CAD build for the part. Positions are in the model's coordinates, mm. A direction names the side the tool comes from. Round coordinates to 2 decimals unless told otherwise and drop trailing zeros. Loops run counter-clockwise (first coordinate to the right, second up) from the corner with the lowest first, then second, coordinate; pieces in that order, holes last. Notation, with made-up numbers: (86.25, 27) - (106.25, 27) arc R21 cw to (106.25, 53) - close; hole circle Ø2 at (-31, 31). An arc over 180 degrees is marked (long way). Use one line per item in the form item = value.
from build123d import *

# Parameters (mm, degrees)
BOSS_EXTRUDE1_DEPTH = 20
FILLET1_R           = 2
CUT_EXTRUDE1_DEPTH  = 76.381086892
CHAMFER1_SIZE       = 0.5
CHAMFER2_SIZE       = 10
CHAMFER3_SIZE       = 1


with BuildPart() as part:
    # Sketch1 → Boss-Extrude1 (new body)
    with BuildSketch(Plane.XY):
        with BuildLine():
            Line((12.7, 20.547), (-12.7, 20.547))
            ThreePointArc((-12.7, 20.547), (-27.228923033, 14.528923033), (-33.247, 0))
            Line((-33.247, 0), (-33.247, -20.447))
            Line((-33.247, -20.447), (-60.015, -20.447))
            Line((-60.015, -20.447), (-60.015, -16.447))
            Line((-60.015, -16.447), (-37.247, -16.447))
            Line((-37.247, -16.447), (-37.247, 0))
            ThreePointArc((-37.247, 0), (-30.057350158, 17.357350158), (-12.7, 24.547))
            Line((-12.7, 24.547), (12.7, 24.547))
            ThreePointArc((12.7, 24.547), (30.057350158, 17.357350158), (37.247, 0))
            Line((37.247, 0), (37.247, -16.447))
            Line((37.247, -16.447), (60.015, -16.447))
            Line((60.015, -16.447), (60.015, -20.447))
            Line((60.015, -20.447), (33.247, -20.447))
            Line((33.247, -20.447), (33.247, 0))
            ThreePointArc((33.247, 0), (27.228923033, 14.528923033), (12.7, 20.547))
        make_face()
    extrude(amount=BOSS_EXTRUDE1_DEPTH)

    # Fillet1
    fillet1_edges = [part.edges().sort_by_distance(p)[0] for p in [
        (60.015, -18.447, 20),
        (-60.015, -18.447, 0),
        (60.015, -18.447, 0),
        (-60.015, -18.447, 20),
    ]]
    fillet(fillet1_edges, radius=FILLET1_R)

    # Sketch3 → Cut-Extrude1 (cut, through all)
    with BuildSketch(Plane(origin=(0, -16.447, 0), x_dir=(1, 0, 0), z_dir=(0, 1, 0))):
        with BuildLine():
            Line((52.015, -2.4), (56.015, -2.4))
            ThreePointArc((56.015, -2.4), (57.615, -4), (56.015, -5.6))
            Line((56.015, -5.6), (52.015, -5.6))
            ThreePointArc((52.015, -5.6), (50.415, -4), (52.015, -2.4))
        make_face()
        with BuildLine():
            Line((56.015, -17.6), (52.015, -17.6))
            ThreePointArc((52.015, -17.6), (50.415, -16), (52.015, -14.4))
            Line((52.015, -14.4), (56.015, -14.4))
            ThreePointArc((56.015, -14.4), (57.615, -16), (56.015, -17.6))
        make_face()
        with BuildLine():
            Line((-52.015, -5.6), (-56.015, -5.6))
            ThreePointArc((-56.015, -5.6), (-57.615, -4), (-56.015, -2.4))
            Line((-56.015, -2.4), (-52.015, -2.4))
            ThreePointArc((-52.015, -2.4), (-50.415, -4), (-52.015, -5.6))
        make_face()
        with BuildLine():
            Line((-56.015, -14.4), (-52.015, -14.4))
            ThreePointArc((-52.015, -14.4), (-50.415, -16), (-52.015, -17.6))
            Line((-52.015, -17.6), (-56.015, -17.6))
            ThreePointArc((-56.015, -17.6), (-57.615, -16), (-56.015, -14.4))
        make_face()
    extrude(amount=-CUT_EXTRUDE1_DEPTH, mode=Mode.SUBTRACT)

    # Chamfer1
    chamfer1_edges = [part.edges().sort_by_distance(p)[0] for p in [
        (-50.415, -20.447, 16),
        (-54.015, -20.447, 17.6),
        (-57.615, -20.447, 16),
        (-54.015, -20.447, 14.4),
        (-50.415, -16.447, 16),
        (-54.015, -16.447, 14.4),
        (-57.615, -16.447, 16),
        (-54.015, -16.447, 17.6),
        (50.415, -20.447, 4),
        (54.015, -20.447, 2.4),
        (57.615, -20.447, 4),
        (54.015, -20.447, 5.6),
        (50.415, -16.447, 4),
        (54.015, -16.447, 5.6),
        (57.615, -16.447, 4),
        (54.015, -16.447, 2.4),
        (57.615, -20.447, 16),
        (54.015, -20.447, 17.6),
        (50.415, -20.447, 16),
        (54.015, -20.447, 14.4),
        (57.615, -16.447, 16),
        (54.015, -16.447, 14.4),
        (50.415, -16.447, 16),
        (54.015, -16.447, 17.6),
        (-50.415, -20.447, 4),
        (-54.015, -20.447, 5.6),
        (-57.615, -20.447, 4),
        (-54.015, -20.447, 2.4),
        (-50.415, -16.447, 4),
        (-54.015, -16.447, 2.4),
        (-57.615, -16.447, 4),
        (-54.015, -16.447, 5.6),
    ]]
    chamfer(chamfer1_edges, length=CHAMFER1_SIZE)

    # Chamfer2
    chamfer2_edges = [part.edges().sort_by_distance(p)[0] for p in [
        (-37.247, -16.447, 10),
        (37.247, -16.447, 10),
    ]]
    chamfer(chamfer2_edges, length=CHAMFER2_SIZE)

    # Chamfer3
    chamfer3_edges = [part.edges().sort_by_distance(p)[0] for p in [
        (0, 20.547, 0),
        (-27.228923033, 14.528923033, 0),
        (-33.247, -10.2235, 0),
        (33.247, -10.2235, 0),
        (27.228923033, 14.528923033, 0),
        (27.228923033, 14.528923033, 20),
        (-33.247, -10.2235, 20),
        (-27.228923033, 14.528923033, 20),
        (0, 20.547, 20),
        (33.247, -10.2235, 20),
    ]]
    chamfer(chamfer3_edges, length=CHAMFER3_SIZE)


solid = part.part
1) Slice it at D-D (x = 44). Write the cut outline in (y, z), plus the area to 3 significant figures.
Report:
outline = (-20.45, 0) - (-13.2, 0) - (-13.2, 20) - (-20.45, 20) - close
area = 145 mm^2
2) Slice it at B-B (y = -14.5). Write the cut outline in (x, z), plus the area to 3 significant figures.
Report:
outline = (-45.3, 0) - (-34.25, 0) - (-33.25, 1) - (-33.25, 19) - (-34.25, 20) - (-45.3, 20) - close; (33.25, 1) - (34.25, 0) - (45.3, 0) - (45.3, 20) - (34.25, 20) - (33.25, 19) - close
area = 480 mm^2
3) Slice it at C-C (y = -9). Write the cut outline in (x, z).
Report:
outline = (-39.8, 0) - (-34.25, 0) - (-33.25, 1) - (-33.25, 19) - (-34.25, 20) - (-39.8, 20) - close; (33.25, 1) - (34.25, 0) - (39.8, 0) - (39.8, 20) - (34.25, 20) - (33.25, 19) - close
4) Two-plate mould, pull along X, no slides. Class faces 1 (the cylindrical face through (-59.445, -18.419, 0.601)), 2 (the flat face through (-54, -16.447, 10)), 3 (the cylindrical face through (59.445, -18.475, 19.399)), 4 (the conical face through (50.28, -16.81, 16.04)): +X half, -X half, draft (parallel to the pull), parting line (faces both ways), or undercut.
Report:
face_1 = -X half
face_2 = draft
face_3 = +X half
face_4 = undercut
5) Tool access for faces 5 (the conical face through (-27.19, 14.81, 19.17)), 6 (the flat face through (54, -18, 14.4)), 7 (the conical face through (50.28, -20.08, 3.96)): list every direction of +Z, -Z, +X, -X, +Y, -Y with a clear straight run to the whole face (end or side of a thin tool).
Report:
face_5 = +Z, -Y
face_6 = +Y, -Y
face_7 = -Y
6) Slice it at A-A (z = 4). State how many separate pieces and enclosed holes the cut face has, plus the area to 3 significant figures.
Report:
separate_pieces = 3
enclosed_holes = 0
area = 772 mm^2
7) Drill centre lines: probe 1 along X at (y, z) = (-4, 6); probe 2 along Y at (x, z) = (-52.5, 6.75); probe 3 along X at (y, z) = (-9.5, 13.5). Where is each one in solid material? Low to high.
Report:
probe_1 = -37.25 to -33.25, 33.25 to 37.25
probe_2 = -20.45 to -16.45
probe_3 = -40.3 to -33.25, 33.25 to 40.3
8) Flat gauge pins, fed straight in: pin 1 (1.9 mm diameter, centred on y = -1.5, z = 12.5, fed in from -X); pin 2 (10 mm diameter, centred on x = 50.5, z = 11, fed in from +Y); pin 3 (5.5 mm diameter, centred on x = -4.5, z = 5.5, fed in from -Y). Where does each tip first touch, or does it go through?
Report:
pin_1 = -37.25
pin_2 = -14.7
pin_3 = 20.55
